Could you check a few things on this model? Use its own coordinates, in mm. A direction names the side the tool comes from. Round coordinates to 2 decimals unless told otherwise and drop trailing zeros. Write each loop counter-clockwise with the first axis right and the second up, starting at its lowest first coordinate (ties: lowest second). Pieces come first, ordered by that corner, then holes. Notation, with made-up numbers: M -34,62.25 L 18,62.25 A20 cw 18,83.25 Z; hole C 0.5,-37 d6. An arc over 180 degrees is marked long. One line per item, written item: value. Start each with the question number.
(1) I'm going to push flat-ended pins straight in: pin 1 Ø6 at (x, z) = (11.5, 20.5) entering from -Y; pin 2 Ø3 at (y, z) = (0, 8.54) entering from -X; pin 3 Ø8 at (x, z) = (17.5, 28) entering from -Y; pin 4 Ø3 at (x, y) = (0, -9.5) entering from +Z. Where does each tip first touch, or does it pass through?
(2) I want a section at A-A on y = 0. Please give me the cut outline in (x, z) (1 decimal).
(3) Which directions (+Z, -Z, +X, -X, +Y, -Y) give clear straight access to the entire face, cutting with the end or side of a thin tool? Please do faces 1 (the face through (22.871, 13.243, 11.765)), 2 (the face through (25.32, -0.9, 19.64)), 3 (the face through (-0.18, -25.87, 8.87)), 4 (the face through (-21.92, 0, 7)).
(4) If I drill on L1, parallel to Y at x = -0.5, z = 31.5; L2, parallel to Z at x = 0, y = -27.5; L3, parallel to Z at x = -13.5, y = -12.5, over which ranges is the centre line in solid material (lowest first)?
(5) I want a section at C-C on z = 20.5. Please give me the cut outline in (x, y) (1 decimal), and give its area (3 significant figures).
(6) I want a section at B-B on x = 0. Count the separate pieces of the cut face and the enclosed holes in it, and give its area (3 significant figures).
(7) Thinking about a two-plate mould opening in Y: for faces 5 (the face through (7, -5, 36.703)), 6 (the face through (0, -26.429, 12)), 7 (the face through (-22.4, 0.1, 1.778)), which applies, released by +Y, released by -Y, zero draft, split by the parting line, or undercut?
```python
from build123d import *

# Parameters (mm, degrees)
BOSS_EXTRUDE1_DEPTH                             = 39.878
BOSS_EXTRUDE2_START                             = -3.175
BOSS_EXTRUDE2_DEPTH                             = 3.175
CBORE_FOR_2_PAN_HEAD_MACHINE_SCREW1_D           = 2.7051
CBORE_FOR_2_PAN_HEAD_MACHINE_SCREW1_DEPTH       = 2.667
CBORE_FOR_2_PAN_HEAD_MACHINE_SCREW1_CBORE_D     = 4.7625
CBORE_FOR_2_PAN_HEAD_MACHINE_SCREW1_CBORE_DEPTH = 1.5748
CBORE_START                                     = 26.4287
CBORE_FOR_2_PAN_HEAD_MACHINE_SCREW2_OUT_R       = 2.38125
CBORE_FOR_2_PAN_HEAD_MACHINE_SCREW2_DEPTH       = 1.574800075
CBORE_START_2                                   = 25.300372244
CBORE_FOR_2_PAN_HEAD_MACHINE_SCREW2_2_O_R       = 1.35255
CBORE_FOR_2_PAN_HEAD_MACHINE_SCREW2_2_DEPTH     = 1.128327756
CBORE_START_3                                   = -28.003500101
CBORE_FOR_2_PAN_HEAD_MACHINE_SCREW3_OUT_R       = 2.38125
CBORE_FOR_2_PAN_HEAD_MACHINE_SCREW3_DEPTH       = 1.574800101
CBORE_START_4                                   = -26.4287
CBORE_FOR_2_PAN_HEAD_MACHINE_SCREW3_2_O_R       = 1.35255
CBORE_FOR_2_PAN_HEAD_MACHINE_SCREW3_2_DEPTH     = 1.128327733
CUT_EXTRUDE1_REACH                              = 58.202
SKETCH20_R                                      = 7.27
HOLE1_AT_2_COUNT                                = 2
HOLE1_AT_2_PITCH                                = 19
F_0_CLEARANCE_HOLE1_D                           = 1.8542
CUT_EXTRUDE2_DEPTH                              = 1.778
CHAMFER1_SIZE                                   = 1.27


# Read off the part's stored shape, not the designer's step: CBORE for #2 Pan Head Machine Screw2, CBORE for #2 Pan Head Machine Screw3
with BuildPart() as part:
    # Sketch1 → Boss-Extrude1 (new body)
    with BuildSketch(Plane.XY):
        with BuildLine():
            Line((-23.495, 15.237486251), (-23.495, -15.237486251))
            ThreePointArc((-23.495, -15.237486251), (28.0035, 0), (-23.495, 15.237486251))
        make_face()
        with BuildLine():
            Line((-20.828, 14.42680312), (-20.828, -14.42680312))
            ThreePointArc((-20.828, -14.42680312), (25.3365, 0), (-20.828, 14.42680312))
        make_face(mode=Mode.SUBTRACT)
    extrude(amount=BOSS_EXTRUDE1_DEPTH)

    # Sketch10 → Boss-Extrude2 (add)
    with BuildSketch(Plane.XY.offset(39.878).offset(BOSS_EXTRUDE2_START)):
        with BuildLine():
            Line((-23.495, 15.237486251), (-23.495, -15.237486251))
            ThreePointArc((-23.495, -15.237486251), (28.0035, 0), (-23.495, 15.237486251))
        make_face()
    extrude(amount=BOSS_EXTRUDE2_DEPTH)

    # CBORE for #2 Pan Head Machine Screw1
    with Locations(Plane(origin=(-23.495, 13.798981486, 10.2108), x_dir=(0, 0, -1), z_dir=(-1, 0, 0))):
        with Locations((1.6708, 13.798981486)):
            CounterBoreHole(CBORE_FOR_2_PAN_HEAD_MACHINE_SCREW1_D / 2, CBORE_FOR_2_PAN_HEAD_MACHINE_SCREW1_CBORE_D / 2, CBORE_FOR_2_PAN_HEAD_MACHINE_SCREW1_CBORE_DEPTH, depth=CBORE_FOR_2_PAN_HEAD_MACHINE_SCREW1_DEPTH)

    # CBORE for #2 Pan Head Machine Screw2 out → CBORE for #2 Pan Head Machine Screw2 (cut)
    with BuildSketch(Plane(origin=(0, 0, 0), x_dir=(0.500000000000004, -0.8660254037844363, 0), z_dir=(0.8660254037844363, 0.5000000000000042, 0)).offset(CBORE_START)):
        with Locations((0, -10.2108)):
            Circle(CBORE_FOR_2_PAN_HEAD_MACHINE_SCREW2_OUT_R)
    extrude(amount=CBORE_FOR_2_PAN_HEAD_MACHINE_SCREW2_DEPTH, mode=Mode.SUBTRACT)

    # CBORE for _2 Pan Head Machine Screw2 2 o → CBORE for _2 Pan Head Machine Screw2 2 (cut)
    with BuildSketch(Plane(origin=(0, 0, 0), x_dir=(0.500000000000004, -0.8660254037844363, 0), z_dir=(0.8660254037844363, 0.5000000000000042, 0)).offset(CBORE_START_2)):
        with Locations((0, -10.2108)):
            Circle(CBORE_FOR_2_PAN_HEAD_MACHINE_SCREW2_2_O_R)
    extrude(amount=CBORE_FOR_2_PAN_HEAD_MACHINE_SCREW2_2_DEPTH, mode=Mode.SUBTRACT)

    # CBORE for #2 Pan Head Machine Screw3 out → CBORE for #2 Pan Head Machine Screw3 (cut)
    with BuildSketch(Plane(origin=(0, 0, 0), x_dir=(1, 0, 0), z_dir=(0, 1, 0)).offset(CBORE_START_3)):
        with Locations((0, -10.2108)):
            Circle(CBORE_FOR_2_PAN_HEAD_MACHINE_SCREW3_OUT_R)
    extrude(amount=CBORE_FOR_2_PAN_HEAD_MACHINE_SCREW3_DEPTH, mode=Mode.SUBTRACT)

    # CBORE for _2 Pan Head Machine Screw3 2 o → CBORE for _2 Pan Head Machine Screw3 2 (cut)
    with BuildSketch(Plane(origin=(0, 0, 0), x_dir=(1, 0, 0), z_dir=(0, 1, 0)).offset(CBORE_START_4)):
        with Locations((0, -10.2108)):
            Circle(CBORE_FOR_2_PAN_HEAD_MACHINE_SCREW3_2_O_R)
    extrude(amount=CBORE_FOR_2_PAN_HEAD_MACHINE_SCREW3_2_DEPTH, mode=Mode.SUBTRACT)

    # Sketch20 → Cut-Extrude1 (cut, up to next)
    with BuildSketch(Plane.XY.offset(39.878), mode=Mode.PRIVATE) as cut_extrude1_sk1:
        Circle(SKETCH20_R)
    cut_extrude1_tool1 = extrude(cut_extrude1_sk1.sketch, amount=-CUT_EXTRUDE1_REACH, mode=Mode.PRIVATE) & part.part
    add(cut_extrude1_tool1.solids().sort_by_distance((0, 0, 39.878))[0], mode=Mode.SUBTRACT)

    # Sketch22 → Hole1 (revolve, cut)
    with BuildSketch(Plane(origin=(0, 9.5, 36.703), x_dir=(0, 1, 0), z_dir=(1, 0, 0))):
        Polygon((0, 0), (0, 2.921), (1.4986, 2.921), (1.6383, 0), align=None)
    hole1 = revolve(axis=Axis((0, 9.5, 146.703), (0, 0, -1)), mode=Mode.SUBTRACT)

    # Hole1 at 2: Hole1 ×2
    with Locations(*[(0, -i * HOLE1_AT_2_PITCH, 0) for i in range(1, HOLE1_AT_2_COUNT)]):
        add(hole1, mode=Mode.SUBTRACT)

    # #0 Clearance Hole1 (through all)
    with Locations(Plane(origin=(0, 0, 36.703), x_dir=(-1, 0, 0), z_dir=(0, 0, -1))):
        with Locations((0, 9.5), (0, -9.5)):
            Hole(F_0_CLEARANCE_HOLE1_D / 2)

    # Sketch25 → Cut-Extrude2 (cut)
    with BuildSketch(Plane(origin=(0, 0, 0), x_dir=(-1, 0, 0), z_dir=(0, 0, -1))):
        with BuildLine():
            Line((23.495, -15.237486251), (23.495, 15.237486251))
            ThreePointArc((23.495, 15.237486251), (-28.0035, 0), (23.495, -15.237486251))
        make_face()
        with BuildLine():
            Line((20.828, -14.42680312), (20.828, 14.42680312))
            ThreePointArc((20.828, 14.42680312), (-25.3365, 0), (20.828, -14.42680312))
        make_face(mode=Mode.SUBTRACT)
    extrude(amount=-CUT_EXTRUDE2_DEPTH, mode=Mode.SUBTRACT)

    # Chamfer1
    chamfer1_edges = [part.edges().sort_by_distance(p)[0] for p in [
        (-20.828, 0, 1.778),
        (25.3365, 0, 1.778),
    ]]
    chamfer(chamfer1_edges, length=CHAMFER1_SIZE)


solid = part.part
```
Found:
1. pin 1: stops at y = -26.68
1. pin 2: stops at x = -21.92
1. pin 3: stops at y = -24.53
1. pin 4: stops at z = 39.88
2. outline: M -23.5,1.8 L -22.1,1.8 L -20.8,3 L -20.8,7.2 L -21.9,7.2 L -21.9,6.2 L -23.5,6.2 Z; M -23.5,10.9 L -21.9,10.9 L -21.9,9.9 L -20.8,9.9 L -20.8,36.7 L -7.3,36.7 L -7.3,39.9 L -23.5,39.9 Z; M 7.3,36.7 L 25.3,36.7 L 25.3,3 L 26.6,1.8 L 28,1.8 L 28,39.9 L 7.3,39.9 Z
3. face 1: none
3. face 2: -Z
3. face 3: -Y
3. face 4: -X
4. L1: y = -28 to -25.33, 25.33 to 28
4. L2: z = 1.78 to 7.83, 12.59 to 39.88
4. L3: z = 36.7 to 39.88
5. outline: M -23.5,-15.2 A28 ccw long -23.5,15.2 Z; hole M -20.8,-14.4 A25.3 ccw long -20.8,14.4 Z
5. area: 442 mm²
6. separate pieces: 5
6. enclosed holes: 0
6. area: 287 mm²
7. face 5: undercut
7. face 6: released by -Y
7. face 7: zero draft
